The listing builds one solid part. Answer for the finished solid, in the listing's coordinates (mm). Face numbers are marked on the shaded views. A direction names the side the tool comes from. Round coordinates to 2 decimals unless told otherwise and drop trailing zeros. Write each loop counter-clockwise with the first axis right and the second up, starting at its lowest first coordinate (ties: lowest second). Pieces come first, ordered by that corner, then holes.
(1) Find the intervals of material crossed by probe 1 along Z at (x, y) = (-9, 7); probe 2 along Z at (x, y) = (-7, 4.25); probe 3 along X at (y, z) = (3.5, -11.5), in increasing order.
(2) The mould has two halves that part along Z. Classify the marked faces 3, 4 and 5: +Z half, -Z half, draft (parallel to the pull), parting line (faces both ways), or undercut.
(3) For the marked faces 1 and 2, determine the directions among +Z, -Z, +X, -X, +Y, -Y from which every point of the face is accessible in a straight line to the end or side of a thin tool.
(4) A cutting plane is placed at D-D, the plane z = 3.5. Give the vertices of the cut face in (x, y).
(5) A cutting plane is placed at A-A, the plane z = 11.5. Give the vertices of the cut face in (x, y).
(6) Each of these flat-tipped pins is pushed along its axis until it touches: pin 1 Ø2.5 at (x, y) = (9.5, 3.5) entering from +Z; pin 2 Ø4 at (y, z) = (3.5, -0.5) entering from +X. Where does it stop, or does it pass through?
(7) A cutting plane is placed at B-B, the plane y = 1.25. Give the vertices of the cut face in (x, z), and give its area (3 significant figures).
(8) A cutting plane is placed at C-C, the plane x = -9. Give the vertices of the cut face in (y, z), and give its area (4 significant figures).
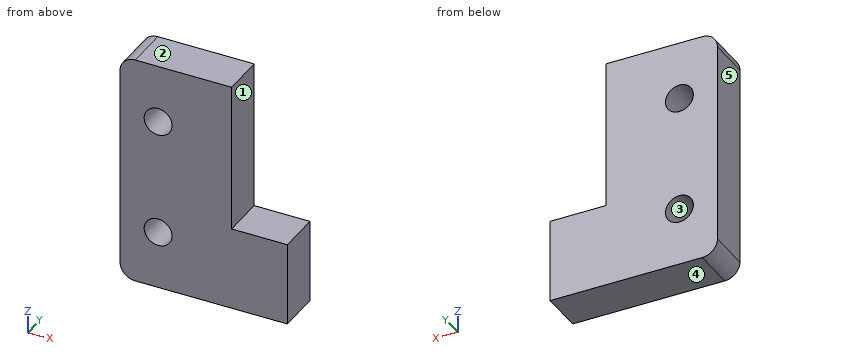
from build123d import *

# Parameters (mm, degrees)
ESBO_O3_R                = 2.75
RESSALTO_EXTRUS_O1_DEPTH = 8.5


with BuildPart() as part:
    # Esboço3 → Ressalto-extrusão1 (new body)
    with BuildSketch(Plane(origin=(0, 0, 0), x_dir=(1, 0, 0), z_dir=(0, 1, 0))):
        with BuildLine():
            Line((-16.5, 20), (-16.5, -20))
            ThreePointArc((-16.5, -20), (-15.621320344, -22.121320344), (-13.5, -23))
            Line((-13.5, -23), (5.5, -23))
            Line((5.5, -23), (5.5, 6.5))
            Line((5.5, 6.5), (16.5, 6.5))
            Line((16.5, 6.5), (16.5, 23))
            Line((16.5, 23), (-13.5, 23))
            ThreePointArc((-13.5, 23), (-15.621320344, 22.121320344), (-16.5, 20))
        make_face()
        with Locations((-9, 11.5)):
            Circle(ESBO_O3_R, mode=Mode.SUBTRACT)
        with Locations((-9, -11.5)):
            Circle(ESBO_O3_R, mode=Mode.SUBTRACT)
    extrude(amount=RESSALTO_EXTRUS_O1_DEPTH)


solid = part.part
Solutions:
1. probe 1: z = -23 to -14.25, -8.75 to 8.75, 14.25 to 23
1. probe 2: z = -23 to -13.39, -9.61 to 9.61, 13.39 to 23
1. probe 3: x = -16.5 to -11.75, -6.25 to 16.5
2. face 3: undercut
2. face 4: -Z half
2. face 5: draft
3. face 1: +Z, +X, +Y, -Y
3. face 2: +Z, +X, -X, +Y, -Y
4. outline: (-16.5, 0) - (5.5, 0) - (5.5, 8.5) - (-16.5, 8.5) - close
5. outline: (-16.5, 0) - (-11.75, 0) - (-11.75, 8.5) - (-16.5, 8.5) - close; (-6.25, 0) - (5.5, 0) - (5.5, 8.5) - (-6.25, 8.5) - close
6. pin 1: stops at z = -6.5
6. pin 2: stops at x = 5.5
7. outline: (-16.5, -20) arc R3 ccw to (-13.5, -23) - (16.5, -23) - (16.5, -6.5) - (5.5, -6.5) - (5.5, 23) - (-13.5, 23) arc R3 ccw to (-16.5, 20) - close; hole circle Ø5.5 at (-9, -11.5); hole circle Ø5.5 at (-9, 11.5)
7. area: 1,140 mm2
8. outline: (0, -23) - (8.5, -23) - (8.5, -14.25) - (0, -14.25) - close; (0, -8.75) - (8.5, -8.75) - (8.5, 8.75) - (0, 8.75) - close; (0, 14.25) - (8.5, 14.25) - (8.5, 23) - (0, 23) - close
8. area: 297.5 mm2
